Read the model definition and answer for the solid it produces. Units are mm, in the model's axes. A direction names the side the tool comes from. Round coordinates to 2 decimals unless told otherwise and drop trailing zeros. Order: outer loops, then holes, each group sorted by start corner. A loop starts at its lowest first (then second) coordinate and runs counter-clockwise, first axis right, second up. Notation, with made-up numbers: M 73.5,37.25 L 85.5,37.25 A20 ccw 85.5,41.25 Z; hole C 80,73 d7. An arc over 180 degrees is marked long. Answer as CSV lines item,"result".
```python
from build123d import *

# Parameters (mm, degrees)
ESBO_O1_W                = 220
ESBO_O1_H                = 145
ESBO_O1_W_2              = 210
ESBO_O1_H_2              = 135
RESSALTO_EXTRUS_O1_DEPTH = 60
ESBO_O3_W                = 210
ESBO_O3_H                = 135
ESBO_O3_R                = 15
RESSALTO_EXTRUS_O3_DEPTH = 1
RESSALTO_EXTRUS_O8_START = -20
ESBO_O14_R               = 15
RESSALTO_EXTRUS_O8_DEPTH = 20
CHANFRO4_SIZE            = 15


with BuildPart() as part:
    # Esboço1 → Ressalto-extrusão1 (new, symmetric)
    with BuildSketch(Plane.XY):
        Rectangle(ESBO_O1_W, ESBO_O1_H)
        Rectangle(ESBO_O1_W_2, ESBO_O1_H_2, mode=Mode.SUBTRACT)
    extrude(amount=RESSALTO_EXTRUS_O1_DEPTH, both=True)

    # Esboço3 → Ressalto-extrusão3 (add)
    with BuildSketch(Plane(origin=(0, 0, -60), x_dir=(-1, 0, 0), z_dir=(0, 0, -1))):
        Rectangle(ESBO_O3_W, ESBO_O3_H)
        Circle(ESBO_O3_R, mode=Mode.SUBTRACT)
    extrude(amount=-RESSALTO_EXTRUS_O3_DEPTH)

    # Esboço14 → Ressalto-extrusão8 (add)
    with BuildSketch(Plane.XY.offset(60).offset(RESSALTO_EXTRUS_O8_START)):
        with BuildLine():
            Line((-20, 0), (-20, -67.5))
            Line((-20, -67.5), (20, -67.5))
            Line((20, -67.5), (20, 0))
            ThreePointArc((20, 0), (0, 20), (-20, 0))
        make_face()
        with Locations(Location((0, 0, 0), (0, 0, 180))):
            Circle(ESBO_O14_R, mode=Mode.SUBTRACT)
    extrude(amount=RESSALTO_EXTRUS_O8_DEPTH)

    # Chanfro4
    chanfro4_edges = [part.edges().sort_by_distance(p)[0] for p in [
        (0, -67.5, 40),
        (20, -67.5, 50),
        (-20, -67.5, 50),
    ]]
    chamfer(chanfro4_edges, length=CHANFRO4_SIZE)


solid = part.part
```
Item 1: A cutting plane is placed at B-B, the plane y = -32. Determine the outline of the cut face in (x, z).
Ans:
outline,"M -110,-60 L 110,-60 L 110,60 L 105,60 L 105,-59 L -105,-59 L -105,60 L -110,60 Z; M -20,40 L 20,40 L 20,60 L -20,60 Z"
Item 2: Flat-ended cylindrical pins translate along their axes: pin 1 (12 mm diameter, centred on x = 9.5, y = 1.5, fed in from -Z); pin 2 (10 mm diameter, centred on x = 44, y = -38, fed in from +Z). Find the tip coordinate at first contact, or state that the pin passes through.
Ans:
pin 1,"z = -60"
pin 2,"z = -59"
Item 3: A cutting plane is placed at D-D, the plane x = -26. Determine the outline of the cut face in (y, z), and give its area (3 significant figures).
Ans:
outline,"M -72.5,-60 L 72.5,-60 L 72.5,60 L 67.5,60 L 67.5,-59 L -67.5,-59 L -67.5,25 L -58.5,34 L -58.5,60 L -72.5,60 Z"
area,"1,610 mm2"
Item 4: A cutting plane is placed at A-A, the plane x = 0. Determine the outline of the cut face in (y, z).
Ans:
outline,"M -72.5,-60 L -15,-60 L -15,-59 L -67.5,-59 L -67.5,25 L -52.5,40 L -15,40 L -15,60 L -72.5,60 Z; M 15,-60 L 72.5,-60 L 72.5,60 L 67.5,60 L 67.5,-59 L 15,-59 Z; M 15,40 L 20,40 L 20,60 L 15,60 Z"
Item 5: A tool of negligible diameter and unlimited length cuts with its end or side. For faces 5 (the face through (-105, -1, 1)), 6 (the face through (14.985, 0.66, -59.507)), 7 (the face through (-0.5, -59.9, 32.6)), from which of +Z, -Z, +X, -X, +Y, -Y can it reach the whole face along a straight path? Write none if from no direction.
Ans:
face 5,"+Z"
face 6,"+Z, -Z"
face 7,"none"
Item 6: Find the intervals of material crossed by probe 1 along Y at (x, z) = (0, 52.5); probe 2 along Y at (x, z) = (-37, 42); probe 3 along X at (y, z) = (47.5, 27), in increasing order. Write a range as [from, to].
Ans:
probe 1,"[-72.5, -15], [15, 20], [67.5, 72.5]"
probe 2,"[-72.5, -67.5], [67.5, 72.5]"
probe 3,"[-110, -105], [105, 110]"
Item 7: Determine the mould class of faces 1 (the face through (-27.4, -59.9, 46.1)), 2 (the face through (-110, -1, 1)), 3 (the face through (-9, -16, 60)), 4 (the face through (1, 16, -59)) for opening direction X: +X half, -X half, draft (parallel to the pull), parting line (faces both ways), or undercut.
Ans:
face 1,"undercut"
face 2,"-X half"
face 3,"draft"
face 4,"undercut"
Item 8: A cutting plane is placed at C-C, the plane z = -38. Determine the outline of the cut face in (x, y), and give its area (3 significant figures).
Ans:
outline,"M -110,-72.5 L 110,-72.5 L 110,72.5 L -110,72.5 Z; hole M -105,-67.5 L 105,-67.5 L 105,67.5 L -105,67.5 Z"
area,"3,550 mm2"
